Model file for the job. Use its own axes, mm. A direction names the side the tool comes from. Coordinates: 2 decimals unless noted, no trailing zeros. Loops run counter-clockwise (first coordinate to the right, second up) from the corner with the lowest first, then second, coordinate; pieces in that order, holes last.
from build123d import *

# Parameters (mm, degrees)
SM_START                 = -3
SM_BASE_FLANGE_1_DEPTH   = 6
CUT_EXTRUDE_1_DEPTH      = 231.181450165
CUT_EXTRUDE_1_DEPTH_BACK = 231.181450165
SKETCH_7_W               = 4
SKETCH_7_H               = 47
CHAMFER_2_SIZE           = 8
CHAMFER_3_SIZE           = 4


# Read off the part's stored shape, not the designer's step: Базовая кромка1
with BuildPart() as part:
    # Базовая кромка1 outline → Базовая кромка1 (new body)
    with BuildSketch(Plane(origin=(0, 0, 0), x_dir=(0, 0, -1), z_dir=(1, 0, 0)).offset(SM_START)):
        with BuildLine():
            Line((-111.5, 0), (-111.5, 146))
            Line((-111.5, 146), (-153.5, 146))
            Line((-153.5, 146), (-153.5, -71.5))
            ThreePointArc((-153.5, -71.5), (-124.210678119, -142.210678119), (-53.5, -171.5))
            Line((-53.5, -171.5), (53.5, -171.5))
            ThreePointArc((53.5, -171.5), (124.210678119, -142.210678119), (153.5, -71.5))
            Line((153.5, -71.5), (153.5, 146))
            Line((153.5, 146), (111.5, 146))
            Line((111.5, 146), (111.5, 0))
            ThreePointArc((111.5, 0), (0, -111.5), (-111.5, 0))
        make_face()
    extrude(amount=SM_BASE_FLANGE_1_DEPTH)

    # Эскиз7 → Вырез-Вытянуть1 (cut, two sides: drawn at the far end of the back side and taken through both)
    with BuildSketch(Plane(origin=(0, 0, 0), x_dir=(0, 0, -1), z_dir=(1, 0, 0)).offset(-CUT_EXTRUDE_1_DEPTH_BACK)):
        with Locations((-113.5, 122.5)):
            Rectangle(SKETCH_7_W, SKETCH_7_H)
        with Locations((113.5, 122.5)):
            Rectangle(SKETCH_7_W, SKETCH_7_H)
    extrude(amount=CUT_EXTRUDE_1_DEPTH + CUT_EXTRUDE_1_DEPTH_BACK, mode=Mode.SUBTRACT)

    # Фаска2
    chamfer_2_edges = [part.edges().sort_by_distance(p)[0] for p in [
        (0, 146, 115.5),
        (0, 146, -115.5),
    ]]
    chamfer(chamfer_2_edges, length=CHAMFER_2_SIZE)

    # Фаска3
    chamfer_3_edges = [part.edges().sort_by_distance(p)[0] for p in [
        (0, 99, -111.5),
        (0, 99, 111.5),
    ]]
    chamfer(chamfer_3_edges, length=CHAMFER_3_SIZE - 0.0001)  # a hair under: the kernel refuses the full size


solid = part.part
Q1. Slice it at A-A (y = -37). List the corners of the cut face in (x, z).
Answers:
outline: (-3, -153.5) - (3, -153.5) - (3, -105.18) - (-3, -105.18) - close; (-3, 105.18) - (3, 105.18) - (3, 153.5) - (-3, 153.5) - close
Q2. Which spindle directions (+Z, -Z, +X, -X, +Y, -Y) get a long thin tool onto all of the face, cutting with end or side? Do faces 1 (the flat face through (3, -116, 2)), 2 (the flat face through (0, 142.1, -119.6)). Say none if no direction does.
Answers:
face 1: +Z, -Z, +X, +Y, -Y
face 2: +X, -X, +Y
Q3. Slice it at C-C (z = 0). List the corners of the cut face in (x, y), and give its area (3 significant figures).
Answers:
outline: (-3, -171.5) - (3, -171.5) - (3, -111.5) - (-3, -111.5) - close
area: 360 mm2
Q4. Slice it at D-D (y = -97). List the corners of the cut face in (x, z).
Answers:
outline: (-3, -150.19) - (3, -150.19) - (3, -54.98) - (-3, -54.98) - close; (-3, 54.98) - (3, 54.98) - (3, 150.19) - (-3, 150.19) - close
Q5. Mould opens along Z. For faces 3 (the flat face through (-3, -116, 2)), 4 (the flat face through (0, 141.9, 119.4)), 5 (the cylindrical face through (-0.042, -141.429, 124.984)), 6 (the cylindrical face through (-0.042, -142.984, -123.429)) say: +Z half, -Z half, draft (parallel to the pull), parting line (faces both ways), or undercut.
Answers:
face 3: draft
face 4: undercut
face 5: +Z half
face 6: -Z half
Q6. Drill centre lines: line 1 (Z direction, x = 2, y = 121); line 2 (Z direction, x = 0.5, y = 93); line 3 (Y direction, x = -0.5, z = 66). Where is each one in solid material? Low to high.
Answers:
line 1: z = -153.5 to -115.5, 115.5 to 153.5
line 2: z = -153.5 to -111.5, 111.5 to 153.5
line 3: y = -170.72 to -89.87
Q7. Flat gauge pin, fed straight in: P1, Ø2, axis at x = 2, z = 111.5, coming from the -Y side. Where does the tip first touch, or does it go through?
Answers:
P1: stops at y = -153.66
